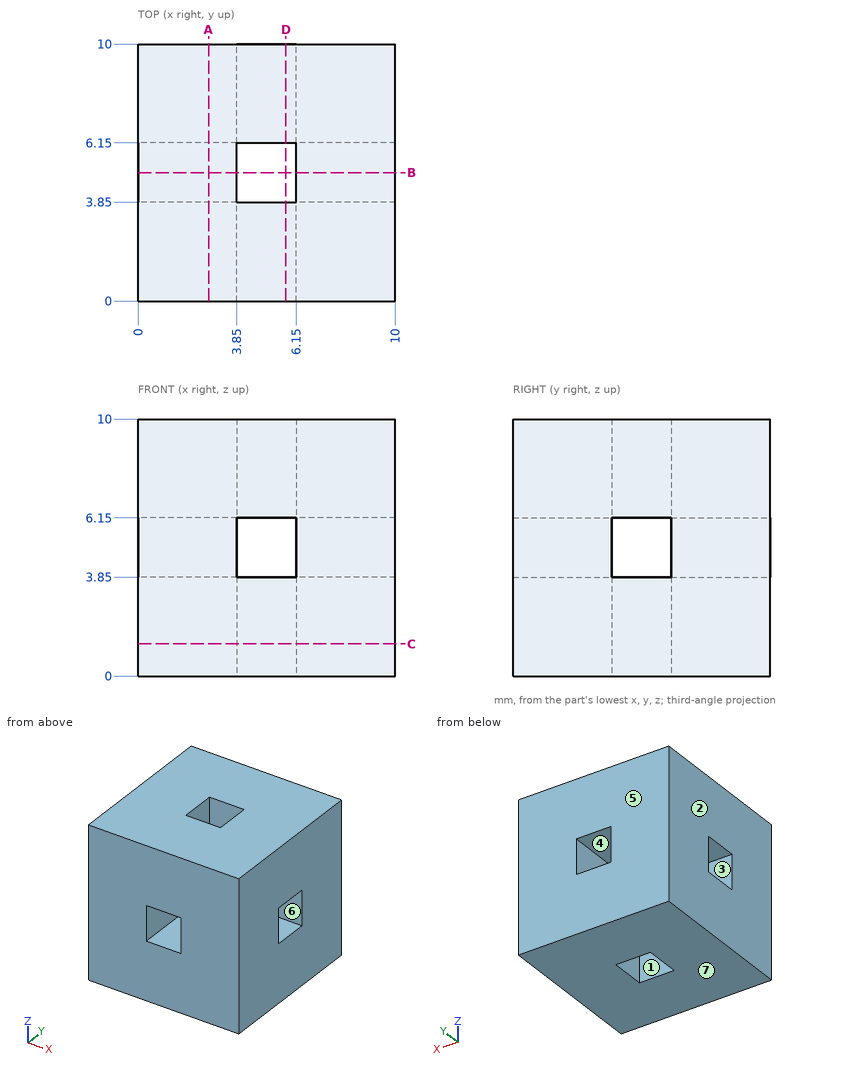
Input: dimensioned drawing with shaded views. Units: mm. Origin: part minimum x, y, z. A direction names the side the tool comes from. Coordinates: 2 decimals unless noted, no trailing zeros. Loops run counter-clockwise (first coordinate to the right, second up) from the corner with the lowest first, then second, coordinate; pieces in that order, holes last. Notation, with made-up numbers: (48, 77) -> (57, 77) arc R17 cw to (57, 107) -> close; hole circle Ø11 at (-11, 68). An arc over 180 degrees is marked (long way). Use a Markdown table: item, result. Add a question column.
(1) Pin query (flat end, axial travel): pin 1 Ø2.5 at (x, y) = (4.5, 8) entering from -Z. Return the tip coordinate at first contact, or that it passes through.
(2) Line query: line 1 along Y through (x, z) = (6.75, 4.75). Output: solid intervals per line, ascending.
(3) Section query B-B, the plane y = 5. Return loops of the section in (x, z).
(4) Access query for the marked faces 1, 2, 3 and 4. Directions: +Z, -Z, +X, -X, +Y, -Y. A direction counts if a zero-diameter tool reaches every point of the face in a straight line with its end or side. Return the directions, or none.
(5) Section query A-A, the plane x = 2.75. Return loops of the section in (y, z).
(6) Mould query, pull axis Z, two halves, no side actions, for the marked faces 5, 6 and 7. Classes: pulls with the +Z half, pulls with the -Z half, needs draft (parallel to the pull), parting line crosses it, or undercut.
Answer:
| question | item | result |
|---|---|---|
| 1 | pin 1 | stops at z = 0 |
| 2 | line 1 | y = 0 to 3.85, 6.15 to 10 |
| 3 | outline | (0, 0) -> (3.85, 0) -> (3.85, 3.85) -> (0, 3.85) -> close; (0, 6.15) -> (3.85, 6.15) -> (3.85, 10) -> (0, 10) -> close; (6.15, 0) -> (10, 0) -> (10, 3.85) -> (6.15, 3.85) -> close; (6.15, 6.15) -> (10, 6.15) -> (10, 10) -> (6.15, 10) -> close |
| 4 | face 1 | +Z, -Z |
| 4 | face 2 | +Z, -Z, -X, +Y, -Y |
| 4 | face 3 | +X, -X |
| 4 | face 4 | +Y, -Y |
| 5 | outline | (0, 0) -> (10, 0) -> (10, 10) -> (0, 10) -> close; hole (3.85, 3.85) -> (6.15, 3.85) -> (6.15, 6.15) -> (3.85, 6.15) -> close |
| 6 | face 5 | needs draft |
| 6 | face 6 | undercut |
| 6 | face 7 | pulls with the -Z half |
